```python
from build123d import *

# Parameters (mm, degrees)
SKETCH2_R           = 15
SKETCH2_R_2         = 1
BOSS_EXTRUDE2_DEPTH = 1.016
SKETCH3_R           = 15
SKETCH3_R_2         = 13.25
SKETCH3_R_3         = 10.25
SKETCH3_R_4         = 9.5
SKETCH3_R_5         = 6.5
SKETCH3_R_6         = 5.5
SKETCH3_R_7         = 2.5
SKETCH3_R_8         = 1.5
BOSS_EXTRUDE4_DEPTH = 1.016
SKETCH5_R           = 15
SKETCH5_R_2         = 13.25
BOSS_EXTRUDE5_DEPTH = 2.032


with BuildPart() as part:
    # Sketch2 → Boss-Extrude2 (new body)
    with BuildSketch(Plane(origin=(0, 0, 0), x_dir=(1, 0, 0), z_dir=(0, 1, 0))):
        with Locations(Location((0, 0, 0), (0, 0, 270))):
            Circle(SKETCH2_R)
        with Locations(Location((0, 0, 0), (0, 0, 270))):
            Circle(SKETCH2_R_2, mode=Mode.SUBTRACT)
        with Locations(Location((4, 0, 0), (0, 0, 270))):
            Circle(SKETCH2_R_2, mode=Mode.SUBTRACT)
        with Locations(Location((8, 0, 0), (0, 0, 270))):
            Circle(SKETCH2_R_2, mode=Mode.SUBTRACT)
    extrude(amount=BOSS_EXTRUDE2_DEPTH)

    # Sketch3 → Boss-Extrude4 (add)
    # profile 1 of 4: a face of its own
    with BuildSketch(Plane(origin=(0, 1.016, 0), x_dir=(1, 0, 0), z_dir=(0, 1, 0))):
        with Locations(Location((0, 0, 0), (0, 0, 270))):
            Circle(SKETCH3_R)
        with Locations(Location((0, 0, 0), (0, 0, 270))):
            Circle(SKETCH3_R_2, mode=Mode.SUBTRACT)
    # profile 2 of 4: a face of its own
    with BuildSketch(Plane(origin=(0, 1.016, 0), x_dir=(1, 0, 0), z_dir=(0, 1, 0))):
        with Locations(Location((0, 0, 0), (0, 0, 270))):
            Circle(SKETCH3_R_3)
        with Locations(Location((0, 0, 0), (0, 0, 270))):
            Circle(SKETCH3_R_4, mode=Mode.SUBTRACT)
    # profile 3 of 4: a face of its own
    with BuildSketch(Plane(origin=(0, 1.016, 0), x_dir=(1, 0, 0), z_dir=(0, 1, 0))):
        with Locations(Location((0, 0, 0), (0, 0, 270))):
            Circle(SKETCH3_R_5)
        with Locations(Location((0, 0, 0), (0, 0, 270))):
            Circle(SKETCH3_R_6, mode=Mode.SUBTRACT)
    # profile 4 of 4: a face of its own
    with BuildSketch(Plane(origin=(0, 1.016, 0), x_dir=(1, 0, 0), z_dir=(0, 1, 0))):
        with Locations(Location((0, 0, 0), (0, 0, 270))):
            Circle(SKETCH3_R_7)
        with Locations(Location((0, 0, 0), (0, 0, 270))):
            Circle(SKETCH3_R_8, mode=Mode.SUBTRACT)
    extrude(amount=BOSS_EXTRUDE4_DEPTH)

    # Sketch5 → Boss-Extrude5 (add)
    with BuildSketch(Plane(origin=(0, 2.032, 0), x_dir=(1, 0, 0), z_dir=(0, 1, 0))):
        with Locations(Location((0, 0, 0), (0, 0, 270))):
            Circle(SKETCH5_R)
        with Locations(Location((0, 0, 0), (0, 0, 270))):
            Circle(SKETCH5_R_2, mode=Mode.SUBTRACT)
    extrude(amount=BOSS_EXTRUDE5_DEPTH)


solid = part.part
```
Geometry: final body of the model. Coordinates: model frame, mm. A direction names the side the tool comes from. Round coordinates to 2 decimals unless told otherwise and drop trailing zeros. Loops run counter-clockwise (first coordinate to the right, second up) from the corner with the lowest first, then second, coordinate; pieces in that order, holes last. Notation, with made-up numbers: (5, 73) -> (14, 73) arc R8 cw to (14, 84) -> close; hole circle Ø5 at (78, -31.75). An arc over 180 degrees is marked (long way). Use one line per item in the form item = value. Start each with the question number.
1) Section B-B on z = 0. Give the number of separate pieces and of enclosed holes in the cut face, then the cut area to 3 significant figures.
2) Section A-A on x = 8. Output: boundary loops of the cut face in (y, z), then the cut area to 3 significant figures.
3) Access query for faces 1 (the flat face through (-3, 0, 0)), 2 (the cylindrical face through (-5.37, 1.52, -1.19)). Directions: +Z, -Z, +X, -X, +Y, -Y. A direction counts if a zero-diameter tool reaches every point of the face in a straight line with its end or side. Return the directions, or none.
4) Draft query along Z for faces 3 (the cylindrical face through (0.66, 2.004, -14.985)), 4 (the flat face through (-6, 1.016, 4)), 5 (the flat face through (-10, 4.064, 9)). Return one class per face: released by +Z, released by -Z, zero draft, split by the parting line, or undercut.
5) First-contact query: P1, Ø3, axis at x = 1.5, z = 8.5, coming from the +Y side; P2, Ø2.5, axis at x = 4, z = 0, coming from the +Y side; P3, Ø1, axis at y = 3.5, z = -8.5, coming from the -X side. Flat tips, straight axial feed; report the tip coordinate or a pass-through.
6) Line query: L1, parallel to X at y = 0.75, z = 0; L2, parallel to Z at x = -7.5, y = 1.1; L3, parallel to X at y = 1.6, z = -8.5. Output: solid intervals per line, ascending.
7) Section C-C on y = 3.35. Output: boundary loops of the cut face in (x, z).
8) Section D-D on x = -11. Output: boundary loops of the cut face in (y, z), then the cut area to 3 significant figures.
Response:
q1.separate_pieces = 4
q1.enclosed_holes = 0
q1.area = 40.6 mm^2
q2.outline = (0, -12.69) -> (4.06, -12.69) -> (4.06, -10.56) -> (1.02, -10.56) -> (1.02, -6.41) -> (2.03, -6.41) -> (2.03, -5.12) -> (1.02, -5.12) -> (1.02, -1) -> (0, -1) -> close; (0, 1) -> (1.02, 1) -> (1.02, 5.12) -> (2.03, 5.12) -> (2.03, 6.41) -> (1.02, 6.41) -> (1.02, 10.56) -> (4.06, 10.56) -> (4.06, 12.69) -> (0, 12.69) -> close
q2.area = 39.3 mm^2
q3.face_1 = +Z, -Z, +X, -X, -Y
q3.face_2 = +Y
q4.face_3 = split by the parting line
q4.face_4 = undercut
q4.face_5 = zero draft
q5.P1 = 2.03
q5.P2 = 1.02
q5.P3 = -12.69
q6.L1 = -15 to -1, 1 to 3, 5 to 7, 9 to 15
q6.L2 = -12.99 to -10.92, -6.99 to -5.83, 5.83 to 6.99, 10.92 to 12.99
q6.L3 = -12.36 to -10.16, -5.73 to -4.24, 4.24 to 5.73, 10.16 to 12.36
q7.outline = circle Ø30 at (0, 0); hole circle Ø26.5 at (0, 0)
q8.outline = (0, -10.2) -> (4.06, -10.2) -> (4.06, -7.39) -> (1.02, -7.39) -> (1.02, 7.39) -> (4.06, 7.39) -> (4.06, 10.2) -> (0, 10.2) -> close
q8.area = 37.9 mm^2
